from build123d import *

# Parameters (mm, degrees)
SKETCH_1_W                 = 5.2
SKETCH_1_H                 = 5.2
EXTRUDE_1_DEPTH            = 1.5
SKETCH_2_W                 = 3.2
SKETCH_2_H                 = 4
SKETCH_2_W_2               = 2
SKETCH_2_H_2               = 3
CUT_EXTRUDE_1_DEPTH        = 1
EXTRUDE_START              = -0.01
SKETCH_3_W                 = 2.7
SKETCH_3_H                 = 0.2
EXTRUDE_2_DEPTH            = 0.31
PATTERN_LINEAR_1_COUNT     = 3
PATTERN_LINEAR_1_PITCH     = 0.5
PATTERN_LINEAR_1_COL_COUNT = 3
PATTERN_LINEAR_1_COL_PITCH = 0.5
MIRROR_START               = -0.01
MIRROR_1_COPY_1_SKETCH_W   = 2.7
MIRROR_1_COPY_1_SKETCH_H   = 0.2
MIRROR_1_COPY_1_DEPTH      = 0.31
MIRROR_1_COPY_2_SKETCH_W   = 2.7
MIRROR_1_COPY_2_SKETCH_H   = 0.2
MIRROR_1_COPY_2_DEPTH      = 0.31
MIRROR_1_COPY_3_SKETCH_W   = 2.7
MIRROR_1_COPY_3_SKETCH_H   = 0.2
MIRROR_1_COPY_3_DEPTH      = 0.31
MIRROR_1_COPY_4_SKETCH_W   = 2.7
MIRROR_1_COPY_4_SKETCH_H   = 0.2
MIRROR_1_COPY_4_DEPTH      = 0.31


with BuildPart() as part:
    # Эскиз1 → Бобышка-Вытянуть1 (new body)
    with BuildSketch(Plane(origin=(0, 0, 0), x_dir=(1, 0, 0), z_dir=(0, 1, 0))):
        Rectangle(SKETCH_1_W, SKETCH_1_H)
    extrude(amount=EXTRUDE_1_DEPTH)

    # Эскиз2 → Вырез-Вытянуть1 (cut)
    with BuildSketch(Plane(origin=(0, 1.5, 0), x_dir=(1, 0, 0), z_dir=(0, 1, 0))):
        Rectangle(SKETCH_2_W, SKETCH_2_H)
        Rectangle(SKETCH_2_W_2, SKETCH_2_H_2, mode=Mode.SUBTRACT)
    extrude(amount=-CUT_EXTRUDE_1_DEPTH, mode=Mode.SUBTRACT)

    # Эскиз3 → Бобышка-Вытянуть2 (add)
    with BuildSketch(Plane(origin=(0, 0, 0), x_dir=(1, 0, 0), z_dir=(0, 1, 0)).offset(EXTRUDE_START)):
        with Locations((-1.75, 0)):
            Rectangle(SKETCH_3_W, SKETCH_3_H)
    extrude_2 = extrude(amount=EXTRUDE_2_DEPTH)

    # Линейный массив1: Бобышка-Вытянуть2 ×3
    with Locations(*[(0, 0, -i * PATTERN_LINEAR_1_PITCH) for i in range(1, PATTERN_LINEAR_1_COUNT)]):
        add(extrude_2)

    # Линейный массив1 col: Бобышка-Вытянуть2 ×3
    with Locations(*[(0, 0, i * PATTERN_LINEAR_1_COL_PITCH) for i in range(1, PATTERN_LINEAR_1_COL_COUNT)]):
        add(extrude_2)

    # Зеркальное отражение1: Бобышка-Вытянуть2 across plane
    add(extrude_2.mirror(Plane(origin=(0, 0, 0), x_dir=(0, 0, 1), z_dir=(1, 0, 0))))

    # Зеркальное отражение1 copy 1 sketch → Зеркальное отражение1 copy 1 (add)
    with BuildSketch(Plane(origin=(0, 0, -0.5), x_dir=(-1, 0, 0), z_dir=(0, 1, 0)).offset(MIRROR_START)):
        with Locations((-1.75, 0)):
            Rectangle(MIRROR_1_COPY_1_SKETCH_W, MIRROR_1_COPY_1_SKETCH_H)
    extrude(amount=MIRROR_1_COPY_1_DEPTH)

    # Зеркальное отражение1 copy 2 sketch → Зеркальное отражение1 copy 2 (add)
    with BuildSketch(Plane(origin=(0, 0, -1), x_dir=(-1, 0, 0), z_dir=(0, 1, 0)).offset(MIRROR_START)):
        with Locations((-1.75, 0)):
            Rectangle(MIRROR_1_COPY_2_SKETCH_W, MIRROR_1_COPY_2_SKETCH_H)
    extrude(amount=MIRROR_1_COPY_2_DEPTH)

    # Зеркальное отражение1 copy 3 sketch → Зеркальное отражение1 copy 3 (add)
    with BuildSketch(Plane(origin=(0, 0, 0.5), x_dir=(-1, 0, 0), z_dir=(0, 1, 0)).offset(MIRROR_START)):
        with Locations((-1.75, 0)):
            Rectangle(MIRROR_1_COPY_3_SKETCH_W, MIRROR_1_COPY_3_SKETCH_H)
    extrude(amount=MIRROR_1_COPY_3_DEPTH)

    # Зеркальное отражение1 copy 4 sketch → Зеркальное отражение1 copy 4 (add)
    with BuildSketch(Plane(origin=(0, 0, 1), x_dir=(-1, 0, 0), z_dir=(0, 1, 0)).offset(MIRROR_START)):
        with Locations((-1.75, 0)):
            Rectangle(MIRROR_1_COPY_4_SKETCH_W, MIRROR_1_COPY_4_SKETCH_H)
    extrude(amount=MIRROR_1_COPY_4_DEPTH)


solid = part.part
The listing builds one solid part. Answer for the finished solid, in the listing's coordinates (mm). A direction names the side the tool comes from. Coordinates: 2 decimals unless noted, no trailing zeros. Order: outer loops, then holes, each group sorted by start corner. A loop starts at its lowest first (then second) coordinate and runs counter-clockwise, first axis right, second up.
Q1. For a pull along X with two mould halves and no side action, classify faces 1 (the face through (0, 1.5, 0)), 2 (the face through (1, 1, 0)) as pulls with the +X half, pulls with the -X half, needs draft (parallel to the pull), parting line crosses it, or undercut.
Q2. A cutting plane is placed at A-A, the plane y = 0.8. Write down the section's boundary in (x, z), and give its area (3 significant figures).
Q3. A cutting plane is placed at D-D, the plane y = 0.4. Write down the section's boundary in (x, z), and give its area (3 significant figures).
Q4. Consider line 1 (X direction, y = 0.8, z = -0.65); line 2 (X direction, y = 0.6, z = -1.8); line 3 (Y direction, x = 2, z = -0.2). Determine where each line is inside the solid, lowest interval first.
Q5. A cutting plane is placed at B-B, the plane x = -0.25. Write down the section's boundary in (y, z).
Q6. Given P1, Ø2, axis at x = -0.5, z = 1.5, coming from the -Y side, flat-ended and moving along its own axis, determine where the tip first touches the part or whether it passes through.
Q7. Which of the six approach directions +Z, -Z, +X, -X, +Y, -Y give full straight-line access (tool end or side, diameter ignored) to faces 3 (the face through (-1, 1, 0)), 4 (the face through (0, 1, -2.6))?
Answers follow:
1. face 1: needs draft
1. face 2: undercut
2. outline: (-2.6, -2.6) - (2.6, -2.6) - (2.6, 2.6) - (-2.6, 2.6) - close; (-1, -1.5) - (1, -1.5) - (1, 1.5) - (-1, 1.5) - close; hole (-1.6, -2) - (1.6, -2) - (1.6, 2) - (-1.6, 2) - close
2. area: 20.2 mm2
3. outline: (-2.6, -2.6) - (2.6, -2.6) - (2.6, 2.6) - (-2.6, 2.6) - close
3. area: 27.0 mm2
4. line 1: x = -2.6 to -1.6, -1 to 1, 1.6 to 2.6
4. line 2: x = -2.6 to -1.6, 1.6 to 2.6
4. line 3: y = 0 to 1.5
5. outline: (0, -2.6) - (1.5, -2.6) - (1.5, -2) - (0.5, -2) - (0.5, -1.5) - (1.5, -1.5) - (1.5, 1.5) - (0.5, 1.5) - (0.5, 2) - (1.5, 2) - (1.5, 2.6) - (0, 2.6) - close
6. P1: stops at y = -0.01
7. face 3: +Y
7. face 4: -Z, +X, -X, +Y, -Y
